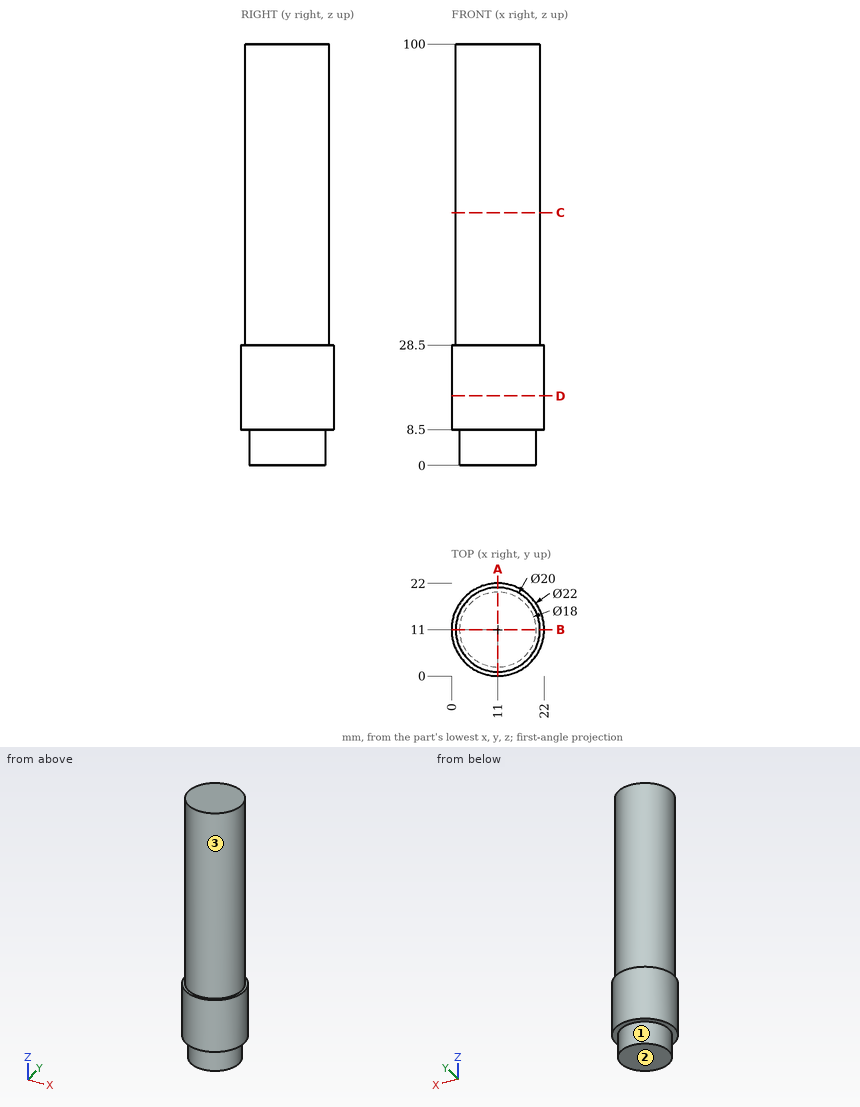
Geometry: see drawing. Coordinates: mm, zero at the bounding-box minimum. A direction names the side the tool comes from. Round coordinates to 2 decimals unless told otherwise and drop trailing zeros. Write each loop counter-clockwise with the first axis right and the second up, starting at its lowest first coordinate (ties: lowest second). Pieces come first, ordered by that corner, then holes. Notation, with made-up numbers: M -34,-5 L 25,-5 A23 ccw 25,17 Z; hole C 78.25,-5 d7. An arc over 180 degrees is marked long. Answer in a Markdown table with one row per item. Add a question column.
(1) Contact query for flat-ended pins moving along their axis: pin 1 (10 mm diameter, centred on y = 6.5, z = 55.5, fed in from -X); pin 2 (4 mm diameter, centred on x = 19.5, z = 87.5, fed in from -Y); pin 3 (4 mm diameter, centred on y = 5.5, z = 57.5, fed in from +X). Output: stop coordinate, or through.
(2) Cut plane D-D, the plane z = 16.5. Return the cut outline in (x, y).
(3) Reachability of the marked faces 1, 2 and 3 from +Z, -Z, +X, -X, +Y, -Y: full face, straight path, thin tool, end or side. Return the list, or none.
(4) Cut plane C-C, the plane z = 60. Return the cut outline in (x, y), then the cut area to 3 significant figures.
(5) Ray query, L1, parallel to Z at x = 20.5, y = 12.75; L2, parallel to Y at x = 7.75, z = 94.5; L3, parallel to Y at x = 17.75, z = 77. Return the intervals inside material, ascending.
(6) Cut plane A-A, the plane x = 11. Return the cut outline in (y, z), then the cut area to 3 significant figures.
Established:
| question | item | result |
|---|---|---|
| 1 | pin 1 | x = 1 |
| 1 | pin 2 | y = 3.4 |
| 1 | pin 3 | x = 20.37 |
| 2 | outline | C 11,11 d22 |
| 3 | face 1 | -Z |
| 3 | face 2 | -Z, +X, -X, +Y, -Y |
| 3 | face 3 | +Z |
| 4 | outline | C 11,11 d20 |
| 4 | area | 314 mm² |
| 5 | L1 | 8.5 to 100 |
| 5 | L2 | 1.54 to 20.46 |
| 5 | L3 | 3.62 to 18.38 |
| 6 | outline | M 0,8.5 L 2,8.5 L 2,0 L 20,0 L 20,8.5 L 22,8.5 L 22,28.5 L 21,28.5 L 21,100 L 1,100 L 1,28.5 L 0,28.5 Z |
| 6 | area | 2,020 mm² |
